from build123d import *

# Parameters (mm, degrees)
SKETCH1_W           = 84
SKETCH1_H           = 104
BOSS_EXTRUDE1_DEPTH = 20
SKETCH2_W           = 82
SKETCH2_H           = 102
CUT_EXTRUDE1_DEPTH  = 5
SKETCH3_W           = 74
SKETCH3_H           = 94
CUT_EXTRUDE2_DEPTH  = 10
SKETCH4_W           = 37.72
SKETCH4_H           = 10
CUT_EXTRUDE4_DEPTH  = 6
SKETCH6_W           = 15
SKETCH6_H           = 10
SKETCH6_W_2         = 10
CUT_EXTRUDE6_DEPTH  = 10
SKETCH7_R           = 1.6
CUT_EXTRUDE7_DEPTH  = 2
SKETCH9_W           = 104
SKETCH9_H           = 10
CUT_EXTRUDE8_DEPTH  = 85


with BuildPart() as part:
    # Sketch1 → Boss-Extrude1 (new body)
    with BuildSketch(Plane(origin=(0, 0, 0), x_dir=(1, 0, 0), z_dir=(0, 1, 0))):
        Rectangle(SKETCH1_W, SKETCH1_H)
    extrude(amount=BOSS_EXTRUDE1_DEPTH)

    # Sketch2 → Cut-Extrude1 (cut)
    with BuildSketch(Plane(origin=(0, 0, 0), x_dir=(-1, 0, 0), z_dir=(0, -1, 0))):
        Rectangle(SKETCH2_W, SKETCH2_H)
    extrude(amount=-CUT_EXTRUDE1_DEPTH, mode=Mode.SUBTRACT)

    # Sketch3 → Cut-Extrude2 (cut)
    with BuildSketch(Plane(origin=(0, 20, 0), x_dir=(1, 0, 0), z_dir=(0, 1, 0))):
        Rectangle(SKETCH3_W, SKETCH3_H)
    extrude(amount=-CUT_EXTRUDE2_DEPTH, mode=Mode.SUBTRACT)

    # Sketch4 → Cut-Extrude4 (cut, through all)
    with BuildSketch(Plane.XY.offset(-47)):
        with Locations((0, 15)):
            Rectangle(SKETCH4_W, SKETCH4_H)
    extrude(amount=-CUT_EXTRUDE4_DEPTH, mode=Mode.SUBTRACT)

    # Sketch6 → Cut-Extrude6 (cut)
    with BuildSketch(Plane(origin=(0, 0, 47), x_dir=(-1, 0, 0), z_dir=(0, 0, -1))):
        with Locations((11.15, 15)):
            Rectangle(SKETCH6_W, SKETCH6_H)
        with Locations((-17.35, 15)):
            Rectangle(SKETCH6_W_2, SKETCH6_H)
    extrude(amount=-CUT_EXTRUDE6_DEPTH, mode=Mode.SUBTRACT)

    # Sketch7 → Cut-Extrude7 (cut)
    with BuildSketch(Plane(origin=(0, 10, 0), x_dir=(1, 0, 0), z_dir=(0, 1, 0))):
        with Locations((18.275, 19)):
            Circle(SKETCH7_R)
        with Locations((-24.825, -31.8)):
            Circle(SKETCH7_R)
        with Locations((22.975, -32.9)):
            Circle(SKETCH7_R)
        with Locations((-9.625, 19)):
            Circle(SKETCH7_R)
    extrude(amount=-CUT_EXTRUDE7_DEPTH, mode=Mode.SUBTRACT)

    # Sketch9 → Cut-Extrude8 (cut, through all)
    with BuildSketch(Plane.ZY.offset(42)):
        with Locations((0, 15)):
            Rectangle(SKETCH9_W, SKETCH9_H)
    extrude(amount=-CUT_EXTRUDE8_DEPTH, mode=Mode.SUBTRACT)


solid = part.part
Geometry check sheet. Reference: the model listing, model coordinates, mm. A direction names the side the tool comes from. Give positions to 0.01 mm unless a question says otherwise; leave off trailing zeros. Write each loop counter-clockwise with the first axis right and the second up, starting at its lowest first coordinate (ties: lowest second). Pieces come first, ordered by that corner, then holes. Notation, with made-up numbers: M 31,28.25 L 54,28.25 A10 cw 54,46.25 Z; hole C 32,30.5 d6. An arc over 180 degrees is marked long. One line per question, with ' | ' between items.
1. Cross-section at D-D (x = -25). Enter the section's corners in (y, z).
Ans:
outline: M 0,-52 L 10,-52 L 10,30.21 L 8,30.21 L 8,33.39 L 10,33.39 L 10,52 L 0,52 L 0,51 L 5,51 L 5,-51 L 0,-51 Z
2. Cross-section at A-A (x = 1.5). Enter the section's corners in (y, z), plus the area to 3 significant figures.
Ans:
outline: M 0,-52 L 10,-52 L 10,52 L 0,52 L 0,51 L 5,51 L 5,-51 L 0,-51 Z | area: 530 mm2
3. Mould release check, pull along X, two halves, no side actions. Record for faces 1 (the face through (-42, 5, 1)), 2 (the face through (23, 8, 33)), 3 (the face through (-1, 5, 52)): released by +X, released by -X, zero draft, split by the parting line, or undercut.
Ans:
face 1: released by -X | face 2: undercut | face 3: zero draft
4. Cross-section at C-C (z = -19). Enter the section's corners in (x, y) (3 decimals), plus the area to 3 significant figures.
Ans:
outline: M -42,0 L -41,0 L -41,5 L 41,5 L 41,0 L 42,0 L 42,10 L 19.875,10 L 19.875,8 L 16.675,8 L 16.675,10 L -8.025,10 L -8.025,8 L -11.225,8 L -11.225,10 L -42,10 Z | area: 417 mm2
5. Cross-section at B-B (z = 36). Enter the section's corners in (x, y).
Ans:
outline: M -42,0 L -41,0 L -41,5 L 41,5 L 41,0 L 42,0 L 42,10 L -42,10 Z
6. Gauge pin test, flat ends, axial feed: pin 1 (1 mm diameter, centred on x = -10, z = -19, fed in from +Y); pin 2 (24.5 mm diameter, centred on x = 13, z = -11, fed in from -Y). Record the tip position at first contact, or that the pin passes through.
Ans:
pin 1: y = 8 | pin 2: y = 5
7. Set-up check for faces 4 (the face through (19.8, 9.01, -19.48)), 5 (the face through (-41, 2, 1)), 6 (the face through (-1, 5, -52)): record each of +Z, -Z, +X, -X, +Y, -Y from which the full face is reachable in a straight line by a thin tool's end or side.
Ans:
face 4: +Y | face 5: -Y | face 6: -Z, +X, -X, +Y, -Y
8. Scan lines: line 1 along X through (y, z) = (4.25, -43); line 2 along Z through (x, y) = (-22.5, 2); line 3 along X through (y, z) = (9.45, 31.8) (3 decimals). Record each from-to range of solid material in increasing order. Write a range as from..to.
Ans:
line 1: -42..-41, 41..42 | line 2: -52..-51, 51..52 | line 3: -42..-26.425, -23.225..21.813, 24.137..42
